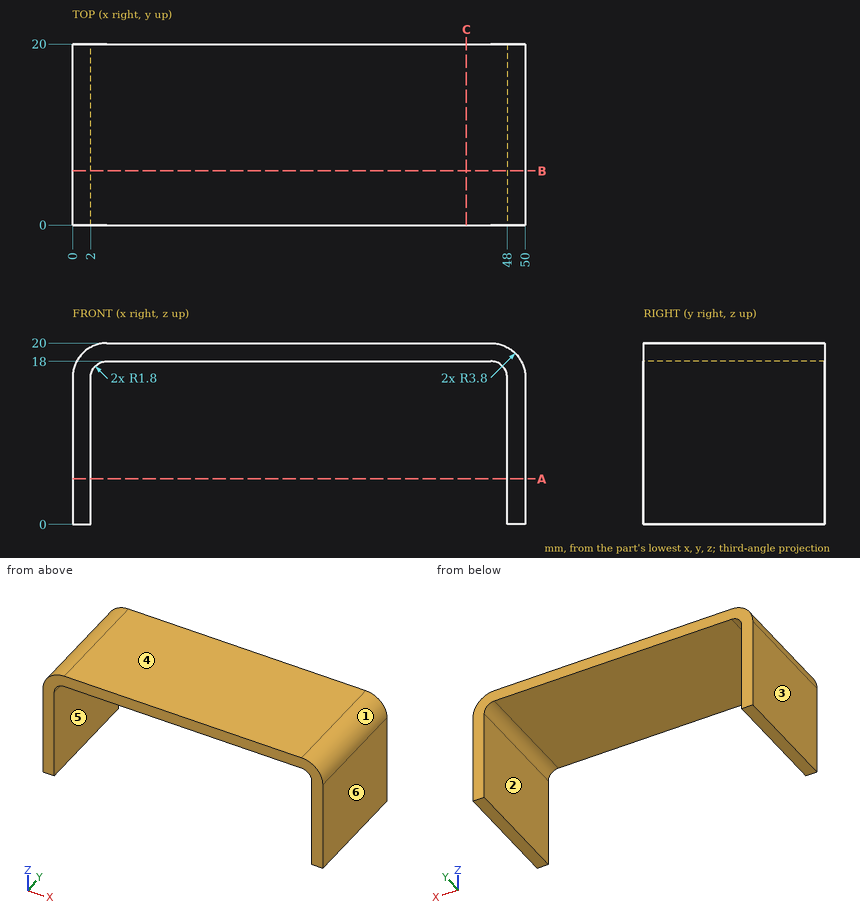
Answer from the drawing. Dimensions are ordinates in mm from the lowest x, y and z of the part. A direction names the side the tool comes from. Coordinates: 2 decimals unless noted, no trailing zeros. Loops run counter-clockwise (first coordinate to the right, second up) from the corner with the lowest first, then second, coordinate; pieces in that order, holes last.
1) Flat-ended cylindrical pins translate along their axes: pin 1 (8 mm diameter, centred on x = 34.5, z = 15, fed in from -Y); pin 2 (10 mm diameter, centred on x = 14, y = 6, fed in from -Z). Find the tip coordinate at first contact, or state that the pin passes through.
Results:
pin 1: stops at y = 0
pin 2: stops at z = 18
2) For a pull along X with two mould halves and no side action, classify the marked faces 1, 2, 3 and 4 as +X half, -X half, draft (parallel to the pull), parting line (faces both ways), or undercut.
Results:
face 1: +X half
face 2: undercut
face 3: -X half
face 4: draft
3) For the marked faces 5 and 6, determine the directions among +Z, -Z, +X, -X, +Y, -Y from which every point of the face is accessible in a straight line to the end or side of a thin tool.
Results:
face 5: -Z, +Y, -Y
face 6: +Z, -Z, +X, +Y, -Y
4) Consider probe 1 along X at (y, z) = (9.25, 7.25); probe 2 along Z at (x, y) = (11, 11.25); probe 3 along X at (y, z) = (11, 17). Determine where each line is inside the solid, lowest interval first.
Results:
probe 1: x = 0 to 2, 48 to 50
probe 2: z = 18 to 20
probe 3: x = 0.09 to 2.19, 47.81 to 49.91
5) Section A-A (z = 5) is taken. Give the vertices of the cut face in (x, y), plus the area to 3 significant figures.
Results:
outline: (0, 0) - (2, 0) - (2, 20) - (0, 20) - close; (48, 0) - (50, 0) - (50, 20) - (48, 20) - close
area: 80.0 mm2
6) Section C-C (x = 43.5) is taken. Give the vertices of the cut face in (y, z), plus the area to 3 significant figures.
Results:
outline: (0, 18) - (20, 18) - (20, 20) - (0, 20) - close
area: 40.0 mm2
7) Section B-B (y = 6) is taken. Give the vertices of the cut face in (x, z), plus the area to 3 significant figures.
Results:
outline: (0, 0) - (2, 0) - (2, 16.2) arc R1.8 cw to (3.8, 18) - (46.2, 18) arc R1.8 cw to (48, 16.2) - (48, 0) - (50, 0) - (50, 16.2) arc R3.8 ccw to (46.2, 20) - (3.8, 20) arc R3.8 ccw to (0, 16.2) - close
area: 167 mm2
